Input: dimensioned drawing with shaded views. Units: mm. Origin: part minimum x, y, z. A direction names the side the tool comes from. Coordinates: 2 decimals unless noted, no trailing zeros. Loops run counter-clockwise (first coordinate to the right, second up) from the corner with the lowest first, then second, coordinate; pieces in that order, holes last. Notation, with made-up numbers: (85, 84) - (101, 84) arc R22 cw to (101, 105) - close; hole circle Ø6 at (66.25, 66.25). An arc over 180 degrees is marked (long way). Put each result on its own line as item: value. Start each with the question number.
1) Section A-A on z = 12.5. Output: boundary loops of the cut face in (x, y) (1 decimal), and give its area (3 significant figures).
2) Material intervals for line 1 along X through (y, z) = (7.75, 5); line 2 along Z through (x, y) = (18, 6) (3 decimals); line 3 along X through (y, z) = (1.5, 7.5), sorted ascending. Write a range as from..to.
3) Reachability of the marked faces 1 and 2 from +Z, -Z, +X, -X, +Y, -Y: full face, straight path, thin tool, end or side. Return the list, or none.
4) Contact query for flat-ended pins moving along their axis: pin 1 Ø0.6 at (y, z) = (7.5, 5.5) entering from -X; pin 2 Ø0.8 at (x, y) = (18.5, 7.5) entering from -Z; pin 3 Ø0.5 at (x, z) = (3, 6) entering from +Y. Output: stop coordinate, or through.
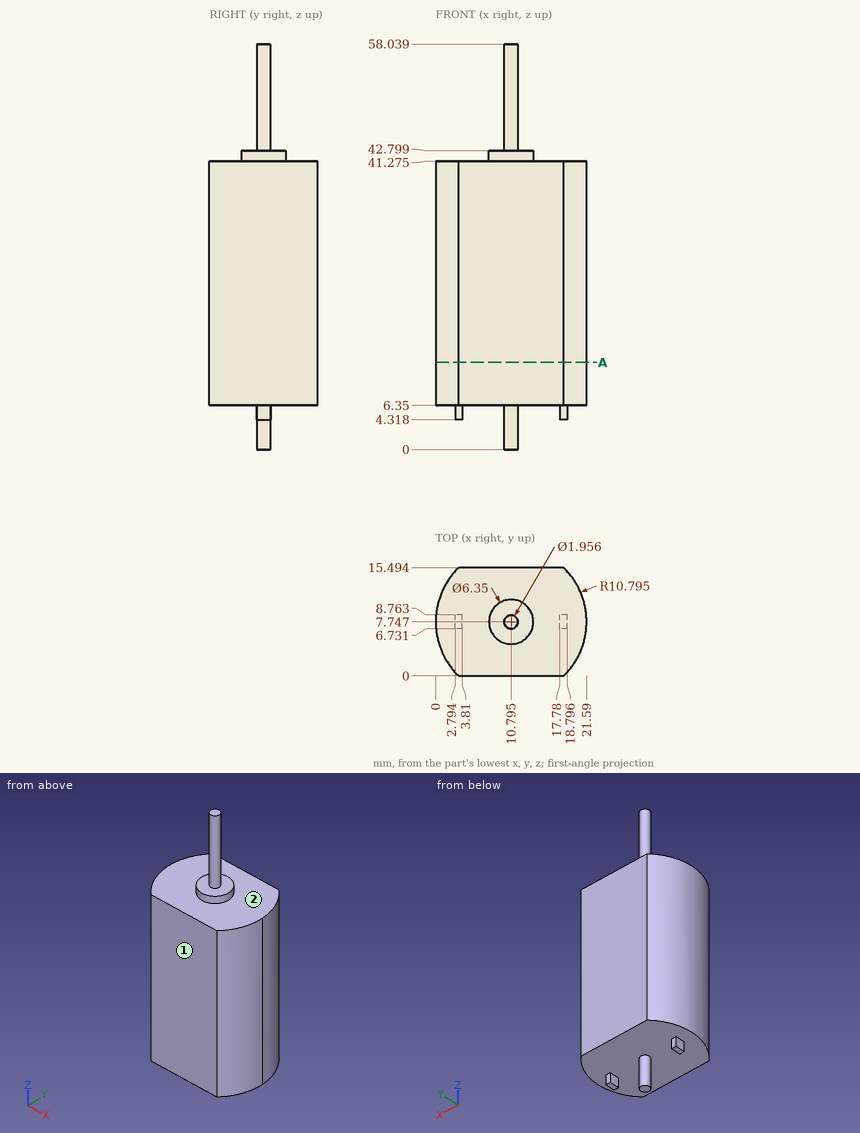
Answer block:
1. outline: (3.3, 0) - (18.3, 0) arc R10.8 ccw to (18.3, 15.5) - (3.3, 15.5) arc R10.8 ccw to start
1. area: 303 mm²
2. line 1: x = 2.79..3.81, 9.82..11.77, 17.78..18.8
2. line 2: z = 6.35..41.275
2. line 3: x = 1.99..19.6
3. face 1: +Z, -Z, +X, -X, -Y
3. face 2: +Z
4. pin 1: stops at x = 2.79
4. pin 2: stops at z = 4.32
4. pin 3: stops at y = 8.76
